from build123d import *

# Parameters (mm, degrees)
SKETCH_1_W               = 108
SKETCH_1_H               = 30
SKETCH_1_W_2             = 10
SKETCH_1_H_2             = 5
EXTRUDE_1_DEPTH          = 6
SKETCH_2_R               = 1.5
CUT_EXTRUDE_1_DEPTH      = 6
SKETCH_3_W               = 94
SKETCH_3_H               = 20
CUT_EXTRUDE_2_DEPTH      = 3
SKETCH_4_R               = 6
EXTRUDE_2_DEPTH          = 3.5
SKETCH_5_R               = 3
CUT_EXTRUDE_3_DEPTH      = 1
SKETCH_6_R               = 1.5
CUT_EXTRUDE_4_DEPTH      = 59.208676329
CUT_EXTRUDE_START        = -3
SKETCH_7_R               = 3
CUT_EXTRUDE_5_DEPTH      = 3
SKETCH_8_R               = 3.5
CUT_EXTRUDE_6_DEPTH      = 1.5
FILLET_1_R               = 1
CUT_EXTRUDE_7_DEPTH      = 111
CUT_EXTRUDE_7_DEPTH_BACK = 111
SKETCH_9_W               = 10
SKETCH_9_H               = 3
SKETCH_10_W              = 13.8
SKETCH_10_H              = 20
EXTRUDE_3_DEPTH          = 3


with BuildPart() as part:
    # 草图1 → 凸台-拉伸1 (new body)
    with BuildSketch(Plane(origin=(0, 0, 0), x_dir=(1, 0, 0), z_dir=(0, 1, 0))):
        Rectangle(SKETCH_1_W, SKETCH_1_H)
        with Locations((-27, 17.5)):
            Rectangle(SKETCH_1_W_2, SKETCH_1_H_2)
        with Locations((27, 17.5)):
            Rectangle(SKETCH_1_W_2, SKETCH_1_H_2)
        with Locations((27, -17.5)):
            Rectangle(SKETCH_1_W_2, SKETCH_1_H_2)
        with Locations((-27, -17.5)):
            Rectangle(SKETCH_1_W_2, SKETCH_1_H_2)
    extrude(amount=EXTRUDE_1_DEPTH)

    # 草图2 → 切除-拉伸1 (cut)
    with BuildSketch(Plane(origin=(0, 6, 0), x_dir=(1, 0, 0), z_dir=(0, 1, 0))):
        with Locations(Location((27, -15, 0), (0, 0, 270))):
            Circle(SKETCH_2_R)
        with Locations(Location((-27, -15, 0), (0, 0, 270))):
            Circle(SKETCH_2_R)
        with Locations(Location((27, 15, 0), (0, 0, 270))):
            Circle(SKETCH_2_R)
        with Locations(Location((-27, 15, 0), (0, 0, 270))):
            Circle(SKETCH_2_R)
    extrude(amount=-CUT_EXTRUDE_1_DEPTH, mode=Mode.SUBTRACT)

    # 草图3 → 切除-拉伸2 (cut)
    with BuildSketch(Plane(origin=(0, 6, 0), x_dir=(1, 0, 0), z_dir=(0, 1, 0))):
        Rectangle(SKETCH_3_W, SKETCH_3_H)
    extrude(amount=-CUT_EXTRUDE_2_DEPTH, mode=Mode.SUBTRACT)

    # 草图4 → 凸台-拉伸2 (add)
    with BuildSketch(Plane.XZ):
        with Locations(Location((-37, 0, 0), (0, 0, 90))):
            Circle(SKETCH_4_R)
        with Locations(Location((37, 0, 0), (0, 0, 90))):
            Circle(SKETCH_4_R)
    extrude(amount=EXTRUDE_2_DEPTH)

    # 草图5 → 切除-拉伸3 (cut)
    with BuildSketch(Plane.XZ.offset(3.5)):
        with Locations(Location((-37, 0, 0), (0, 0, 270))):
            Circle(SKETCH_5_R)
        with Locations(Location((37, 0, 0), (0, 0, 90))):
            Circle(SKETCH_5_R)
    extrude(amount=-CUT_EXTRUDE_3_DEPTH, mode=Mode.SUBTRACT)

    # 草图6 → 切除-拉伸4 (cut, through all)
    with BuildSketch(Plane.XZ.offset(2.5)):
        with Locations(Location((-37, 0, 0), (0, 0, 270))):
            Circle(SKETCH_6_R)
        with Locations(Location((37, 0, 0), (0, 0, 270))):
            Circle(SKETCH_6_R)
    extrude(amount=-CUT_EXTRUDE_4_DEPTH, mode=Mode.SUBTRACT)

    # 草图7 → 切除-拉伸5 (cut)
    with BuildSketch(Plane(origin=(0, 3, 0), x_dir=(1, 0, 0), z_dir=(0, 1, 0)).offset(CUT_EXTRUDE_START)):
        with Locations(Location((-37, 0, 0), (0, 0, 90))):
            Circle(SKETCH_7_R)
        with Locations(Location((37, 0, 0), (0, 0, 270))):
            Circle(SKETCH_7_R)
    extrude(amount=CUT_EXTRUDE_5_DEPTH, mode=Mode.SUBTRACT)

    # 草图8 → 切除-拉伸6 (cut)
    with BuildSketch(Plane(origin=(0, 6, 0), x_dir=(1, 0, 0), z_dir=(0, 1, 0))):
        with Locations(Location((-27, 15, 0), (0, 0, 270))):
            Circle(SKETCH_8_R)
        with Locations(Location((27, 15, 0), (0, 0, 90))):
            Circle(SKETCH_8_R)
        with Locations(Location((27, -15, 0), (0, 0, 270))):
            Circle(SKETCH_8_R)
        with Locations(Location((-27, -15, 0), (0, 0, 90))):
            Circle(SKETCH_8_R)
    extrude(amount=-CUT_EXTRUDE_6_DEPTH, mode=Mode.SUBTRACT)

    # 圆角1
    fillet_1_edges = [part.edges().sort_by_distance(p)[0] for p in [
        (-54, 3, 15),
        (-54, 3, -15),
        (-32, 3, -15),
        (-32, 3, -20),
        (-22, 3, -20),
        (-22, 3, -15),
        (22, 3, -15),
        (22, 3, -20),
        (32, 3, -20),
        (32, 3, -15),
        (54, 3, -15),
        (54, 3, 15),
        (32, 3, 15),
        (32, 3, 20),
        (22, 3, 20),
        (22, 3, 15),
        (-22, 3, 15),
        (-22, 3, 20),
        (-32, 3, 15),
    ]]
    fillet(fillet_1_edges, radius=FILLET_1_R)

    # 草图9 → 切除-拉伸7 (cut, two sides: drawn at the far end of the back side and taken through both)
    with BuildSketch(Plane.ZY.offset(54).offset(-CUT_EXTRUDE_7_DEPTH_BACK)):
        with Locations((0, 4.5)):
            Rectangle(SKETCH_9_W, SKETCH_9_H)
    extrude(amount=CUT_EXTRUDE_7_DEPTH + CUT_EXTRUDE_7_DEPTH_BACK, mode=Mode.SUBTRACT)

    # 草图10 → 凸台-拉伸3 (add)
    with BuildSketch(Plane(origin=(0, 3, 0), x_dir=(1, 0, 0), z_dir=(0, 1, 0))):
        Rectangle(SKETCH_10_W, SKETCH_10_H)
    extrude(amount=EXTRUDE_3_DEPTH)


solid = part.part
For this review, take the finished solid that the model builds, in its own axes (mm). A direction names the side the tool comes from. Round coordinates to 2 decimals unless told otherwise and drop trailing zeros. Write each loop counter-clockwise with the first axis right and the second up, starting at its lowest first coordinate (ties: lowest second). Pieces come first, ordered by that corner, then holes. Notation, with made-up numbers: (75.5, -2.75) - (110.5, -2.75) arc R19 ccw to (110.5, 29.25) - close; hole circle Ø8 at (36.25, 17.5). An arc over 180 degrees is marked (long way). Write item = value, one per line. Start each with the question number.
1. For pin 1 Ø5 at (x, y) = (-47.5, 2.5) entering from -Z; pin 2 Ø4 at (x, z) = (-11.5, 12) entering from -Y; pin 3 Ø1.5 at (y, z) = (1.5, 17.5) entering from +X, all flat-tipped, find the tip position at first contact; note any pin that passes through.
2. Consider section D-D on z = -9. State the section outline as (x, y) points, plus the area to 3 significant figures.
3. For faces 1 (the face through (-47, 5, 8)), 2 (the face through (-22, 3, 18)), 3 (the face through (-32, 3, 18)), 4 (the face through (51, 4, 5)), list the 3-axis set-ups (+Z, -Z, +X, -X, +Y, -Y) from which the entire face can be reached by the end or side of a thin tool; tool diameter is ignored.
4. Wall thickness on L1, parallel to X at y = -3.2, z = 0; L2, parallel to Y at x = 41.5, z = 6; L3, parallel to Z at x = 25, y = 3.25: over which ranges is each line inside the solid? List them lowest first.
5. Consider section A-A on x = 27. State the section outline as (y, z) points, plus the area to 3 significant figures.
6. Consider section B-B on y = -1. State the section outline as (x, z) points, plus the area to 3 significant figures.
7. Draft analysis for pull direction Y (two halves, no side actions). For faces 5 (the face through (38.3, -2.5, 1.3)), 6 (the face through (-54, 2, 0)), 7 (the face through (29, 4.5, -15)), state which applies: released by +Y, released by -Y, zero draft, split by the parting line, or undercut.
8. Consider section C-C on x = -37. State the section outline as (y, z) points.
Evaluation:
q1.pin_1 = -15
q1.pin_2 = 0
q1.pin_3 = 32
q2.outline = (-54, 0) - (54, 0) - (54, 6) - (47, 6) - (47, 3) - (6.9, 3) - (6.9, 6) - (-6.9, 6) - (-6.9, 3) - (-47, 3) - (-47, 6) - (-54, 6) - close
q2.area = 407 mm2
q3.face_1 = +Y
q3.face_2 = +Z, +Y, -Y
q3.face_3 = +Z, -X, +Y, -Y
q3.face_4 = +X, +Y
q4.L1 = -43 to -40, -34 to -31, 31 to 34, 40 to 43
q4.L2 = 0 to 3
q4.L3 = -20 to -10, 10 to 20
q5.outline = (0, -20) - (6, -20) - (6, -18.5) - (4.5, -18.5) - (4.5, -16.5) - (0, -16.5) - close; (0, -13.5) - (4.5, -13.5) - (4.5, -11.5) - (6, -11.5) - (6, -10) - (3, -10) - (3, 10) - (6, 10) - (6, 11.5) - (4.5, 11.5) - (4.5, 13.5) - (0, 13.5) - close; (0, 16.5) - (4.5, 16.5) - (4.5, 18.5) - (6, 18.5) - (6, 20) - (0, 20) - close
q5.area = 132 mm2
q6.outline = circle Ø12 at (-37, 0); circle Ø12 at (37, 0); hole circle Ø3 at (-37, 0); hole circle Ø3 at (37, 0)
q6.area = 212 mm2
q7.face_5 = released by -Y
q7.face_6 = zero draft
q7.face_7 = released by +Y
q8.outline = (-3.5, -6) - (0, -6) - (0, -15) - (6, -15) - (6, -10) - (3, -10) - (3, -3) - (0, -3) - (0, -1.5) - (-2.5, -1.5) - (-2.5, -3) - (-3.5, -3) - close; (-3.5, 3) - (-2.5, 3) - (-2.5, 1.5) - (0, 1.5) - (0, 3) - (3, 3) - (3, 10) - (6, 10) - (6, 15) - (0, 15) - (0, 6) - (-3.5, 6) - close
